Design review of the part shown in the three views and the two pictorial views. Dimensions are in mm from the part's minimum x, y and z. A direction names the side the tool comes from. Coordinates: 2 decimals unless noted, no trailing zeros. Loops run counter-clockwise (first coordinate to the right, second up) from the corner with the lowest first, then second, coordinate; pieces in that order, holes last. Notation, with made-up numbers: (16, -22.5) - (57, -22.5) arc R31 ccw to (57, 6.5) - close; hole circle Ø3 at (-20.5, 23.25). An arc over 180 degrees is marked (long way). One line per item, written item: value. Start each with the question number.
1. Take a section at C-C, the plane x = 33.5. State the section outline as (y, z) points, and give its area (3 significant figures).
2. For the marked faces 1 and 2, list the 3-axis set-ups (+Z, -Z, +X, -X, +Y, -Y) from which the entire face can be reached by the end or side of a thin tool; tool diameter is ignored.
3. Take a section at A-A, the plane y = 3.5. State the section outline as (x, z) points.
4. The part is to be moulded in two halves that separate along X. For the marked faces 3 and 4, say which applies: released by +X, released by -X, zero draft, split by the parting line, or undercut.
5. Insertion check: pin 1 (3 mm diameter, centred on x = 42.5, y = 18.5, fed in from +Z); pin 2 (1 mm diameter, centred on x = 29.5, z = 1.5, fed in from -Y). Each pin has a flat end and moves straight along its axis. Give the tip position at first contact, or say it passes through.
6. Take a section at B-B, the plane z = 0.7. State the section outline as (x, y) points, and give its area (3 significant figures).
7. To check wall thickness, follow line 1 (X direction, y = 18.75, z = 3.65); line 2 (Y direction, x = 36, z = 4.8). State the ranges of each line that lie inside material, in increasing order. Write a range as from..to.
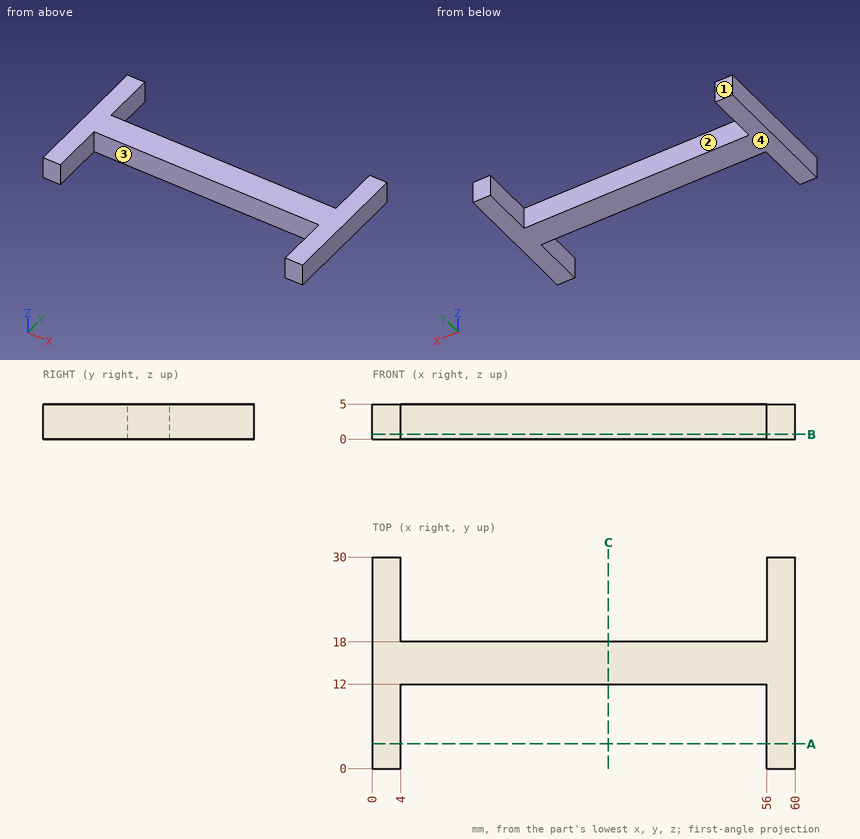
Solutions:
1. outline: (12, 0) - (18, 0) - (18, 5) - (12, 5) - close
1. area: 30.0 mm2
2. face 1: +Z, -Z, +X, -X, +Y
2. face 2: +Z, -Z, +Y
3. outline: (0, 0) - (4, 0) - (4, 5) - (0, 5) - close; (56, 0) - (60, 0) - (60, 5) - (56, 5) - close
4. face 3: undercut
4. face 4: zero draft
5. pin 1: z = 5
5. pin 2: y = 12
6. outline: (0, 0) - (4, 0) - (4, 12) - (56, 12) - (56, 0) - (60, 0) - (60, 30) - (56, 30) - (56, 18) - (4, 18) - (4, 30) - (0, 30) - close
6. area: 552 mm2
7. line 1: 0..4, 56..60
7. line 2: 12..18
